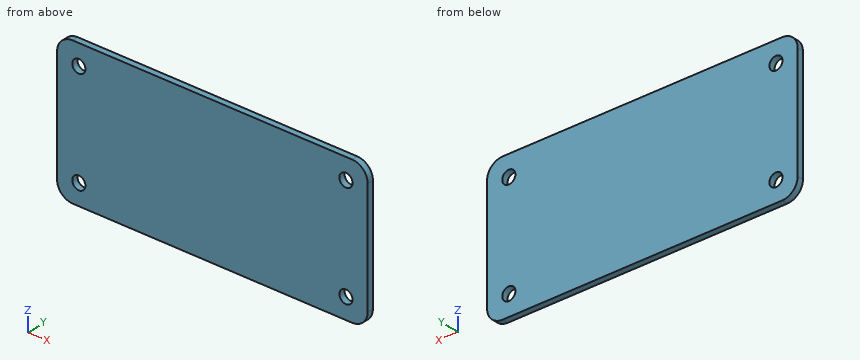
from build123d import *

# Parameters (mm, degrees)
ESBO_O2_W                = 150
ESBO_O2_H                = 70
RESSALTO_EXTRUS_O1_DEPTH = 3
ESBO_O4_R                = 3.175
CORTE_EXTRUS_O1_DEPTH    = 3
FILETE1_R                = 7.5


with BuildPart() as part:
    # Esboço2 → Ressalto-extrusão1 (new body)
    with BuildSketch(Plane(origin=(0, 0, 0), x_dir=(1, 0, 0), z_dir=(0, 1, 0))):
        with Locations((75, 35)):
            Rectangle(ESBO_O2_W, ESBO_O2_H)
    extrude(amount=RESSALTO_EXTRUS_O1_DEPTH)

    # Esboço4 → Corte-extrusão1 (cut)
    with BuildSketch(Plane(origin=(0, 3, 0), x_dir=(1, 0, 0), z_dir=(0, 1, 0))):
        with Locations(Location((10.5, 60, 0), (0, 0, 270))):
            Circle(ESBO_O4_R)
        with Locations(Location((139.5, 60, 0), (0, 0, 270))):
            Circle(ESBO_O4_R)
        with Locations(Location((139.5, 10, 0), (0, 0, 270))):
            Circle(ESBO_O4_R)
        with Locations(Location((10.5, 10, 0), (0, 0, 270))):
            Circle(ESBO_O4_R)
    extrude(amount=-CORTE_EXTRUS_O1_DEPTH, mode=Mode.SUBTRACT)

    # Filete1
    filete1_edges = [part.edges().sort_by_distance(p)[0] for p in [
        (0, 1.5, -70),
        (150, 1.5, -70),
        (150, 1.5, 0),
        (0, 1.5, 0),
    ]]
    fillet(filete1_edges, radius=FILETE1_R)


solid = part.part
Here's how the part is built. I have some questions about the finished solid (model axes, mm). Coordinates: 2 decimals unless noted, no trailing zeros. Loops run counter-clockwise (first coordinate to the right, second up) from the corner with the lowest first, then second, coordinate; pieces in that order, holes last. Notation, with made-up numbers: (-16.75, -20) -> (4.25, -20) arc R30 ccw to (4.25, 16) -> close; hole circle Ø2 at (2, 23.5). An arc over 180 degrees is marked (long way). Use one line per item in the form item = value. Start each with the question number.
(1) If we section it at A-A (z = -60): Please give me the cut outline in (x, y) (3 decimals), then the cut area to 3 significant figures.
(2) If we section it at C-C (x = 10.5): Please give me the cut outline in (y, z) (3 decimals), then the cut area to 3 significant figures.
(3) If we section it at B-B (y = 1): Please give me the cut outline in (x, z) (3 decimals), then the cut area to 3 significant figures.
(4) Please list where these lines run through material, in increasing order: line 1 along X through (y, z) = (0.7, -10) (3 decimals); line 2 along Z through (x, y) = (13, 0.7); line 3 along X through (y, z) = (0.4, -59.5).
Verdict:
q1.outline = (0, 0) -> (7.325, 0) -> (7.325, 3) -> (0, 3) -> close; (13.675, 0) -> (136.325, 0) -> (136.325, 3) -> (13.675, 3) -> close; (142.675, 0) -> (150, 0) -> (150, 3) -> (142.675, 3) -> close
q1.area = 412 mm²
q2.outline = (0, -70) -> (3, -70) -> (3, -63.175) -> (0, -63.175) -> close; (0, -56.825) -> (3, -56.825) -> (3, -13.175) -> (0, -13.175) -> close; (0, -6.825) -> (3, -6.825) -> (3, 0) -> (0, 0) -> close
q2.area = 172 mm²
q3.outline = (0, -62.5) arc R7.5 ccw to (7.5, -70) -> (142.5, -70) arc R7.5 ccw to (150, -62.5) -> (150, -7.5) arc R7.5 ccw to (142.5, 0) -> (7.5, 0) arc R7.5 ccw to (0, -7.5) -> close; hole circle Ø6.35 at (10.5, -60); hole circle Ø6.35 at (10.5, -10); hole circle Ø6.35 at (139.5, -60); hole circle Ø6.35 at (139.5, -10)
q3.area = 10,300 mm²
q4.line_1 = 0 to 7.325, 13.675 to 136.325, 142.675 to 150
q4.line_2 = -70 to -61.96, -58.04 to -11.96, -8.04 to 0
q4.line_3 = 0 to 7.36, 13.64 to 136.36, 142.64 to 150
